Source: three-view drawing plus pictorial views. Frame: mm from the lowest corner of the part. Round coordinates to 2 decimals unless told otherwise and drop trailing zeros. Loops run counter-clockwise (first coordinate to the right, second up) from the corner with the lowest first, then second, coordinate; pieces in that order, holes last. Notation, with made-up numbers: (52.25, -30.5) -> (66.25, -30.5) arc R14 cw to (66.25, -25.5) -> close; hole circle Ø5 at (53, 82.25). An arc over 180 degrees is marked (long way). Answer in a Markdown table with one row per item.
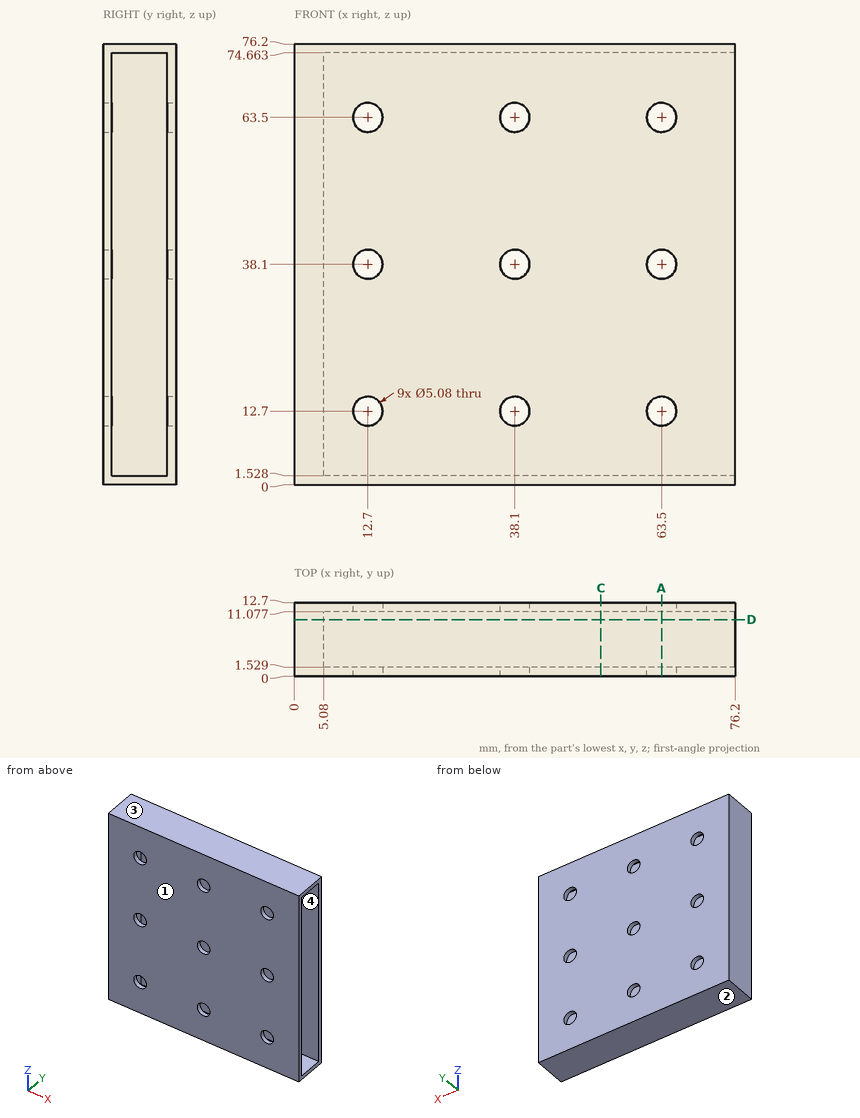
Item 1: Line query: probe 1 along X at (y, z) = (11.9, 38.1); probe 2 along Y at (x, z) = (60, 67.5). Output: solid intervals per line, ascending. Write a range as [from, to].
Answer:
| item | result |
|---|---|
| probe 1 | x = [0, 10.16], [15.24, 35.56], [40.64, 60.96], [66.04, 76.2] |
| probe 2 | y = [0, 1.53], [11.08, 12.7] |
Item 2: Cut plane C-C (x = 53). Output: boundary loops of the cut face in (y, z).
Answer:
| item | result |
|---|---|
| outline | (0, 0) -> (12.7, 0) -> (12.7, 76.2) -> (0, 76.2) -> close; hole (1.53, 1.53) -> (11.08, 1.53) -> (11.08, 74.66) -> (1.53, 74.66) -> close |
Item 3: Draft query along Z for the marked faces 1, 2, 3 and 4. Return one class per face: pulls with the +Z half, pulls with the -Z half, needs draft (parallel to the pull), parting line crosses it, or undercut.
Answer:
| item | result |
|---|---|
| face 1 | needs draft |
| face 2 | pulls with the -Z half |
| face 3 | pulls with the +Z half |
| face 4 | undercut |
Item 4: Cut plane A-A (x = 63.5). Count the separate pieces of the cut face and the enclosed holes in it.
Answer:
| item | result |
|---|---|
| separate pieces | 6 |
| enclosed holes | 0 |
Item 5: Pin query (flat end, axial travel): pin 1 Ø3 at (y, z) = (11, 28) entering from -X; pin 2 Ø3 at (y, z) = (5.5, 60.5) entering from +X. Return the tip coordinate at first contact, or that it passes through.
Answer:
| item | result |
|---|---|
| pin 1 | stops at x = 0 |
| pin 2 | stops at x = 5.08 |
Item 6: Cut plane D-D (y = 9.75). Output: boundary loops of the cut face in (x, z), then the cut area to 3 significant figures.
Answer:
| item | result |
|---|---|
| outline | (0, 0) -> (76.2, 0) -> (76.2, 1.53) -> (5.08, 1.53) -> (5.08, 74.66) -> (76.2, 74.66) -> (76.2, 76.2) -> (0, 76.2) -> close |
| area | 605 mm² |
